Work out the finished part from the listing and answer in its coordinate system (mm). Face numbers are marked on the shaded views. A direction names the side the tool comes from. Round coordinates to 2 decimals unless told otherwise and drop trailing zeros. Loops run counter-clockwise (first coordinate to the right, second up) from the corner with the lowest first, then second, coordinate; pieces in that order, holes last. Notation, with made-up numbers: M 33,-29 L 74,-29 A13 ccw 74,-15 Z; hole C 59,11 d4. An arc over 180 degrees is marked long. One line per item, written item: value.
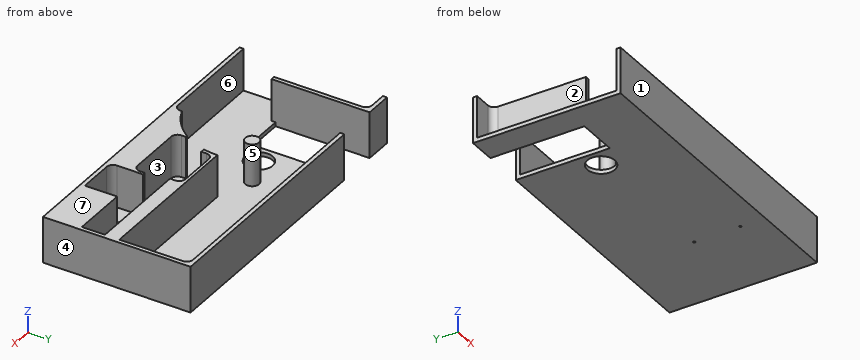
```python
from build123d import *

# Parameters (mm, degrees)
F1_DEPTH  = 25
F2_T      = -2.2
F3_R      = 7.5
F4_DEPTH  = 25
F5_R      = 3.75
F6_DEPTH  = 22.8
F7_W      = 35
F7_H      = 17.5
F8_DEPTH  = 22.8
F9_W      = 24.2
F9_H      = 51
F10_DEPTH = 22.8
F11_W     = 27.0332266644
F11_H     = 1.5
F11_W_2   = 6.9575315177
F11_W_3   = 1.9967853452
F12_DEPTH = 22.8
F13_R     = 3.4
F14_R     = 0.5301707608
F15_DEPTH = 25
F16_W     = 58.4967853452
F16_H     = 7.8
F16_W_2   = 30.5156996727
F16_H_2   = 17.5
F17_DEPTH = 22.8
F18_W     = 5.6
F18_H     = 75.6
F19_DEPTH = 22.8


with BuildPart() as f1:
    # F0 (on Top) → F1 (new body)
    with BuildSketch(Plane.XY):
        Polygon((-70, 40), (-85, 40), (-85, -40), (85, -40), (85, 40), (-48, 40), (-48, -11), (-70, -11), align=None)
    extrude(amount=F1_DEPTH)

    # F2
    f2_openings = [f1.faces().sort_by_distance(p)[0] for p in [
        (5.305177, -1.303815, 25),
    ]]
    offset(amount=F2_T, openings=f2_openings, kind=Kind.INTERSECTION)

    # F3 (on face) → F4 (cut)
    with BuildSketch(Plane.XY.offset(2.2)):
        with Locations((-38, 0)):
            Circle(F3_R)
    extrude(amount=-F4_DEPTH, mode=Mode.SUBTRACT)

    # F5 (on face) → F6 (join, through all)
    with BuildSketch(Plane.XY.offset(2.2)):
        with Locations((-21.3, 6.8)):
            Circle(F5_R)
    extrude(amount=F6_DEPTH)

    # F7 (on face) → F8 (join, through all)
    with BuildSketch(Plane.XY.offset(2.2)):
        with Locations((12.5, -29.05)):
            Rectangle(F7_W, F7_H)
        with BuildLine():
            Line((-5, -20.3), (-8.2693760577, -20.3))
            ThreePointArc((-8.2693760577, -20.3), (-15.628025883, -28.2045169096), (-25, -33.5708206632))
            Line((-25, -33.5708206632), (-25, -37.8))
            Line((-25, -37.8), (-5, -37.8))
            Line((-5, -37.8), (-5, -20.3))
        make_face()
        with BuildLine():
            Line((28.1302789037, 0), (-2, 0))
            ThreePointArc((-2, 0), (-2.2144278138, -3.9233688725), (-2.8551568505, -7.8))
            Line((-2.8551568505, -7.8), (29.5341439003, -7.8))
            ThreePointArc((29.5341439003, -7.8), (28.1976713274, -4.0142062307), (28.1302789037, 0))
        make_face()
    extrude(amount=F8_DEPTH)

    # F9 (on face) → F10 (cut, through all)
    with BuildSketch(Plane.XY.offset(25)):
        with Locations((-57.9, 12.3)):
            Rectangle(F9_W, F9_H)
    extrude(amount=-F10_DEPTH, mode=Mode.SUBTRACT)

    # F11 (on face) → F12 (cut, through all)
    with BuildSketch(Plane.XY.offset(25)):
        with BuildLine():
            Line((-0.5300120096, -6.3), (26.5032146548, -6.3))
            Line((26.5032146548, -6.3), (26.5032146548, -2.1))
            ThreePointArc((26.5032146548, -2.1), (26.5, -1.8), (26.5032146548, -1.5))
            Line((26.5032146548, -1.5), (-0.5300120096, -1.5))
            Line((-0.5300120096, -1.5), (-0.5300120096, -6.3))
        make_face()
        with Locations((12.9866013226, -7.05)):
            Rectangle(F11_W, F11_H)
        with Locations((12.9866013226, -21.05)):
            Rectangle(F11_W, F11_H)
        Polygon((28.5, -21.8), (26.5032146548, -21.8), (-0.5300120096, -21.8), (-7.4875435273, -21.8), (-7.4875435273, -26.3), (28.5, -26.3), align=None)
        with Locations((-4.0087777684, -21.05)):
            Rectangle(F11_W_2, F11_H)
        with Locations((27.5016073274, -21.05)):
            Rectangle(F11_W_3, F11_H)
    extrude(amount=-F12_DEPTH, mode=Mode.SUBTRACT)

    # F13
    f13_edges = [f1.edges().sort_by_distance(p)[0] for p in [
        (-0.530012, -1.5, 13.6),
        (26.503215, -1.5, 13.6),
        (26.503215, -2.1, 13.6),
        (28.5, -26.3, 13.6),
        (-7.487544, -26.3, 13.6),
        (30, -37.8, 13.6),
        (82.8, -37.8, 13.6),
        (82.8, 37.8, 13.6),
        (-72.2, 37.8, 13.6),
        (-82.8, 37.8, 13.6),
        (-82.8, -37.8, 13.6),
        (-25, -37.8, 13.6),
    ]]
    fillet(f13_edges, radius=F13_R)

    # F14 (on face) → F15 (cut)
    with BuildSketch(Plane.XY.offset(2.2)):
        with Locations((40.2, -1.5)):
            Circle(F14_R)
        with Locations((40.2, -26.5)):
            Circle(F14_R)
    extrude(amount=-F15_DEPTH, mode=Mode.SUBTRACT)

    # F16 (on face) → F17 (join, through all)
    with BuildSketch(Plane.XY.offset(25)):
        with Locations((55.7516073274, -3.9)):
            Rectangle(F16_W, F16_H)
        with Locations((67.5421501637, -29.05)):
            Rectangle(F16_W_2, F16_H_2)
    extrude(amount=-F17_DEPTH)

    # F18 (on face) → F19 (cut, through all)
    with BuildSketch(Plane.XY.offset(25)):
        with Locations((-82.2, 0)):
            Rectangle(F18_W, F18_H)
    extrude(amount=-F19_DEPTH, mode=Mode.SUBTRACT)


solid = f1.part
```
1) Find the intervals of material crossed by probe 1 along Y at (x, z) = (5, 20.75); probe 2 along Y at (x, z) = (40.2, 0.55); probe 3 along X at (y, z) = (32, 17), in increasing order. Write a range as from..to.
Check values:
probe 1: -40..-26.3, -1.5..0, 37.8..40
probe 2: -40..-27.03, -25.97..-2.03, -0.97..40
probe 3: -72.2..-70, 82.8..85
2) Find section B-B (x = -38). Give the vertices of the cut face in (y, z).
Check values:
outline: M -40,0 L -7.5,0 L -7.5,2.2 L -37.8,2.2 L -37.8,25 L -40,25 Z; M 7.5,0 L 40,0 L 40,25 L 37.8,25 L 37.8,2.2 L 7.5,2.2 Z
3) Find section C-C (z = 23.25). Give the number of separate pieces and of enclosed holes in the cut face, then the cut area to 3 significant figures.
Check values:
separate pieces: 3
enclosed holes: 0
area: 2,680 mm2
4) Find section D-D (y = -31.5). Give the vertices of the cut face in (x, z).
Check values:
outline: M -85,0 L 85,0 L 85,25 L 52.28,25 L 52.28,2.2 L 30,2.2 L 30,25 L -20.57,25 L -20.57,2.2 L -85,2.2 Z
5) Each of these flat-tipped pins is pushed along its axis until it touches: pin 1 (2.5 mm diameter, centred on y = -6.5, z = 8.5, fed in from -X); pin 2 (8 mm diameter, centred on x = 14, y = -7.5, fed in from +Z); pin 3 (1.8 mm diameter, centred on x = -61, z = 1.5, fed in from +Y); pin 4 (2 mm diameter, centred on x = -48.5, y = 9, fed in from -Z). Where does it stop, or does it pass through?
Check values:
pin 1: x = -72.2
pin 2: z = 2.2
pin 3: y = -11
pin 4: z = 0
6) Find section A-A (y = 24). Give the vertices of the cut face in (x, z), then the cut area to 3 significant figures.
Check values:
outline: M -85,0 L -70,0 L -70,25 L -72.2,25 L -72.2,2.2 L -85,2.2 Z; M -48,0 L 85,0 L 85,25 L 82.8,25 L 82.8,2.2 L -48,2.2 Z
area: 426 mm2
7) The mould has two halves that part along X. Classify the marked faces 1, 2, 3 and 4: +X half, -X half, draft (parallel to the pull), parting line (faces both ways), or undercut.
Check values:
face 1: draft
face 2: -X half
face 3: undercut
face 4: +X half
8) For the marked faces 5, 6 and 7, determine the directions among +Z, -Z, +X, -X, +Y, -Y from which every point of the face is accessible in a straight line to the end or side of a thin tool.
Check values:
face 5: +Z
face 6: +Z, -X
face 7: +Z, +X, -X, +Y, -Y
